Model file for the job. Use its own axes, mm. A direction names the side the tool comes from. Coordinates: 2 decimals unless noted, no trailing zeros. Order: outer loops, then holes, each group sorted by start corner. A loop starts at its lowest first (then second) coordinate and runs counter-clockwise, first axis right, second up. Notation, with made-up numbers: (70.25, 68) -> (74.25, 68) arc R22 ccw to (74.25, 74) -> close; hole circle Ø4 at (-37.5, -33). An arc over 180 degrees is marked (long way). Return JSON: item names as keys, results as strings. Group by question number.
1) Pull direction X, two halves, no side cores. Call faces 4 (the flat face through (-15, 1, 5)), 5 (the flat face through (11.9, 4, 5)), 6 (the flat face through (4.4, 4, 7)): +X half, -X half, draft (parallel to the pull), parting line (faces both ways), or undercut.
2) Flat gauge pins, fed straight in: pin 1 (3 mm diameter, centred on x = -6, z = 5.5, fed in from +Y); pin 2 (4.5 mm diameter, centred on y = 6, z = 3, fed in from -X); pin 3 (0.9 mm diameter, centred on x = 6.5, y = 4.5, fed in from +Z). Where does each tip first touch, or does it go through?
3) Cut at D-D (x = 4.75). Write the cut outline in (y, z).
4) Cut at B-B (y = 8). Write the cut outline in (x, z).
5) Cut at A-A (z = 8). Write the cut outline in (x, y), and give its area (3 significant figures).
6) Probe line 1 (X direction, y = 7.5, z = 3.5); line 2 (X direction, y = 1, z = 6.5); line 3 (Y direction, x = -11.75, z = 4). List the from-to ranges inside material, lowest first.
7) Cut at C-C (y = 2.5). Write the cut outline in (x, z), and give its area (3 significant figures).
8) Which spindle directions (+Z, -Z, +X, -X, +Y, -Y) get a long thin tool onto all of the face, cutting with end or side? Do faces 1 (the flat face through (0, 6, 5)), 2 (the flat face through (10, 4, 10.8)), 3 (the flat face through (7.5, 4, 7)). Say none if no direction does.
from build123d import *

# Parameters (mm, degrees)
SKETCH001_W  = 15
SKETCH001_H  = 10.8
PAD_DEPTH    = 3
PAD001_DEPTH = 8.4


with BuildPart() as part:
    # Sketch001 → Pad (new body)
    with BuildSketch(Plane.XZ):
        with Locations((-7.5, 5.4)):
            Rectangle(SKETCH001_W, SKETCH001_H)
    extrude(amount=-PAD_DEPTH)

    # Sketch → Pad001 (join)
    with BuildSketch(Plane.XZ):
        Polygon((0, 0), (0, 10.8), (4.4, 10.8), (4.4, 3.1), (7.5, 3.1), (7.5, 10.8), (11.9, 10.8), (11.9, 0), align=None)
    extrude(amount=-PAD001_DEPTH)


solid = part.part
Answers below:
{
 "1": {"face 4": "-X half", "face 5": "+X half", "face 6": "undercut"},
 "2": {"pin 1": "stops at y = 3", "pin 2": "stops at x = 0", "pin 3": "stops at z = 3.1"},
 "3": {"outline": "(0, 0) -> (8.4, 0) -> (8.4, 3.1) -> (0, 3.1) -> close"},
 "4": {"outline": "(0, 0) -> (11.9, 0) -> (11.9, 10.8) -> (7.5, 10.8) -> (7.5, 3.1) -> (4.4, 3.1) -> (4.4, 10.8) -> (0, 10.8) -> close"},
 "5": {"outline": "(-15, 0) -> (4.4, 0) -> (4.4, 8.4) -> (0, 8.4) -> (0, 3) -> (-15, 3) -> close; (7.5, 0) -> (11.9, 0) -> (11.9, 8.4) -> (7.5, 8.4) -> close", "area": "119 mm^2"},
 "6": {"line 1": "x = 0 to 4.4, 7.5 to 11.9", "line 2": "x = -15 to 4.4, 7.5 to 11.9", "line 3": "y = 0 to 3"},
 "7": {"outline": "(-15, 0) -> (11.9, 0) -> (11.9, 10.8) -> (7.5, 10.8) -> (7.5, 3.1) -> (4.4, 3.1) -> (4.4, 10.8) -> (-15, 10.8) -> close", "area": "267 mm^2"},
 "8": {"face 1": "+Z, -Z, -X, +Y", "face 2": "+Z, +X, -X, +Y, -Y", "face 3": "+Z, +Y, -Y"}
}
